```python
from build123d import *

# Parameters (mm, degrees)
F0_W     = 25
F0_H     = 283.3333333333
F1_DEPTH = 25


with BuildPart() as f1:
    # F0 (on Front) → F1 (new body)
    with BuildSketch(Plane.XZ):
        Polygon((0, 500), (0, 0), (25, 25), (25, 308.3333333333), (25, 333.3333333333), (25, 351.5717982238), (25, 456.7615351095), (25, 475), align=None)
        Polygon((500, 500), (0, 500), (25, 475), (42.1656140146, 475), (141.1677193187, 475), (158.3333333333, 475), (183.3333333333, 475), (200.4989473479, 475), (299.5010526521, 475), (316.6666666667, 475), (341.6666666667, 475), (358.8322806813, 475), (457.8343859854, 475), (475, 475), align=None)
        Polygon((475, 25), (500, 0), (500, 500), (475, 475), (475, 456.7615351095), (475, 351.5717982238), (475, 333.3333333333), (475, 308.3333333333), align=None)
        Polygon((25, 25), (0, 0), (500, 0), (475, 25), (452.5, 25), (427.5, 25), (405, 25), (380, 25), (357.5, 25), (332.5, 25), (310, 25), (285, 25), (262.5, 25), (237.5, 25), (215, 25), (190, 25), (167.5, 25), (142.5, 25), (120, 25), (95, 25), (72.5, 25), (47.5, 25), align=None)
        Polygon((25, 351.5717982238), (25, 333.3333333333), (42.1656140146, 333.3333333333), (91.6666666667, 385.9282017762), (74.5010526521, 404.1666666667), align=None)
        Polygon((42.1656140146, 475), (25, 475), (25, 456.7615351095), (74.5010526521, 404.1666666667), (91.6666666667, 385.9282017762), (141.1677193187, 333.3333333333), (158.3333333333, 333.3333333333), (158.3333333333, 351.5717982238), (108.8322806813, 404.1666666667), (91.6666666667, 422.4051315572), align=None)
        Polygon((158.3333333333, 475), (141.1677193187, 475), (91.6666666667, 422.4051315572), (108.8322806813, 404.1666666667), (158.3333333333, 456.7615351095), align=None)
        Polygon((183.3333333333, 475), (158.3333333333, 475), (158.3333333333, 456.7615351095), (158.3333333333, 351.5717982238), (158.3333333333, 333.3333333333), (183.3333333333, 333.3333333333), (183.3333333333, 351.5717982238), (183.3333333333, 456.7615351095), align=None)
        Polygon((200.4989473479, 475), (183.3333333333, 475), (183.3333333333, 456.7615351095), (232.8343859854, 404.1666666667), (250, 385.9282017762), (299.5010526521, 333.3333333333), (316.6666666667, 333.3333333333), (316.6666666667, 351.5717982238), (267.1656140146, 404.1666666667), (250, 422.4051315572), align=None)
        Polygon((183.3333333333, 351.5717982238), (183.3333333333, 333.3333333333), (200.4989473479, 333.3333333333), (250, 385.9282017762), (232.8343859854, 404.1666666667), align=None)
        Polygon((316.6666666667, 456.7615351095), (316.6666666667, 475), (299.5010526521, 475), (250, 422.4051315572), (267.1656140146, 404.1666666667), align=None)
        Polygon((341.6666666667, 456.7615351095), (341.6666666667, 475), (316.6666666667, 475), (316.6666666667, 456.7615351095), (316.6666666667, 351.5717982238), (316.6666666667, 333.3333333333), (341.6666666667, 333.3333333333), (341.6666666667, 351.5717982238), align=None)
        Polygon((457.8343859854, 333.3333333333), (475, 333.3333333333), (475, 351.5717982238), (425.4989473479, 404.1666666667), (408.3333333333, 422.4051315572), (358.8322806813, 475), (341.6666666667, 475), (341.6666666667, 456.7615351095), (391.1677193187, 404.1666666667), (408.3333333333, 385.9282017762), align=None)
        Polygon((475, 456.7615351095), (475, 475), (457.8343859854, 475), (408.3333333333, 422.4051315572), (425.4989473479, 404.1666666667), align=None)
        Polygon((341.6666666667, 333.3333333333), (358.8322806813, 333.3333333333), (408.3333333333, 385.9282017762), (391.1677193187, 404.1666666667), (341.6666666667, 351.5717982238), align=None)
        Polygon((25, 333.3333333333), (25, 308.3333333333), (47.5, 308.3333333333), (72.5, 308.3333333333), (95, 308.3333333333), (120, 308.3333333333), (142.5, 308.3333333333), (167.5, 308.3333333333), (190, 308.3333333333), (215, 308.3333333333), (237.5, 308.3333333333), (262.5, 308.3333333333), (285, 308.3333333333), (310, 308.3333333333), (332.5, 308.3333333333), (357.5, 308.3333333333), (380, 308.3333333333), (405, 308.3333333333), (427.5, 308.3333333333), (452.5, 308.3333333333), (475, 308.3333333333), (475, 333.3333333333), (457.8343859854, 333.3333333333), (358.8322806813, 333.3333333333), (341.6666666667, 333.3333333333), (316.6666666667, 333.3333333333), (299.5010526521, 333.3333333333), (200.4989473479, 333.3333333333), (183.3333333333, 333.3333333333), (158.3333333333, 333.3333333333), (141.1677193187, 333.3333333333), (42.1656140146, 333.3333333333), align=None)
        with Locations((60, 166.6666666667)):
            Rectangle(F0_W, F0_H)
        with Locations((107.5, 166.6666666667)):
            Rectangle(F0_W, F0_H)
        with Locations((155, 166.6666666667)):
            Rectangle(F0_W, F0_H)
        with Locations((202.5, 166.6666666667)):
            Rectangle(F0_W, F0_H)
        with Locations((250, 166.6666666667)):
            Rectangle(F0_W, F0_H)
        with Locations((297.5, 166.6666666667)):
            Rectangle(F0_W, F0_H)
        with Locations((345, 166.6666666667)):
            Rectangle(F0_W, F0_H)
        with Locations((392.5, 166.6666666667)):
            Rectangle(F0_W, F0_H)
        with Locations((440, 166.6666666667)):
            Rectangle(F0_W, F0_H)
    extrude(amount=-F1_DEPTH)


solid = f1.part
```
For this review, take the finished solid that the model builds, in its own axes (mm). Coordinates: 2 decimals unless noted, no trailing zeros. Order: outer loops, then holes, each group sorted by start corner. A loop starts at its lowest first (then second) coordinate and runs counter-clockwise, first axis right, second up. Notation, with made-up numbers: (8.5, 18.25) -> (67.5, 18.25) arc R34 cw to (67.5, 48.25) -> close; hole circle Ø5 at (50, 0). An arc over 180 degrees is marked (long way). Use CSV: the item, a comma, the result in double quotes. Start each with the question number.
Item 1: We need section A-A, the plane x = 277. Give the boundary of the cut face in (y, z), then the cut area to 3 significant figures.
Item 2: Draft analysis for pull direction X (two halves, no side actions). For faces 1 (the face through (275.097, 12.325, 449.071)), 2 (the face through (475, 12, 405)), state which applies: pulls with the +X half, pulls with the -X half, needs draft (parallel to the pull), parting line crosses it, or undercut.
Item 3: We need section C-C, the plane x = 444. Give the boundary of the cut face in (y, z).
Item 4: We need section B-B, the plane z = 292. Give the number of separate pieces and of enclosed holes in the cut face, then the cut area to 4 significant figures.
Item 5: Wall thickness on probe 1 along Z at (x, y) = (383, 16); probe 2 along Z at (x, y) = (297.5, 21); probe 3 along Z at (x, y) = (139, 7): over which ranges is each line inside the solid? List them lowest first.
Derived:
1,outline,"(0, 0) -> (25, 0) -> (25, 25) -> (0, 25) -> close; (0, 308.33) -> (25, 308.33) -> (25, 333.33) -> (0, 333.33) -> close; (0, 357.24) -> (25, 357.24) -> (25, 393.72) -> (0, 393.72) -> close; (0, 414.62) -> (25, 414.62) -> (25, 451.09) -> (0, 451.09) -> close; (0, 475) -> (25, 475) -> (25, 500) -> (0, 500) -> close"
1,area,"3,700 mm^2"
2,face 1,"undercut"
2,face 2,"undercut"
3,outline,"(0, 0) -> (25, 0) -> (25, 333.33) -> (0, 333.33) -> close; (0, 348.03) -> (25, 348.03) -> (25, 384.51) -> (0, 384.51) -> close; (0, 423.82) -> (25, 423.82) -> (25, 460.3) -> (0, 460.3) -> close; (0, 475) -> (25, 475) -> (25, 500) -> (0, 500) -> close"
4,separate pieces,"11"
4,enclosed holes,"0"
4,area,"6,875 mm^2"
5,probe 1,"z = 0 to 333.33, 359.01 to 395.49, 412.84 to 449.32, 475 to 500"
5,probe 2,"z = 0 to 333.33, 335.46 to 371.94, 436.4 to 472.87, 475 to 500"
5,probe 3,"z = 0 to 25, 308.33 to 333.33, 335.64 to 372.11, 436.22 to 472.7, 475 to 500"
